Geometry check sheet. Reference: the model listing, model coordinates, mm. A direction names the side the tool comes from. Give positions to 0.01 mm unless a question says otherwise; leave off trailing zeros. Loops run counter-clockwise (first coordinate to the right, second up) from the corner with the lowest first, then second, coordinate; pieces in that order, holes last. Notation, with made-up numbers: (28.25, 35.5) -> (36.25, 35.5) arc R29 ccw to (36.25, 64.5) -> close; hole circle Ø5 at (8, 32.25). An arc over 180 degrees is marked (long way). One line per item, written item: value. Start each with the question number.
(1) Gauge pin test, flat ends, axial feed: pin 1 Ø3 at (x, z) = (-11, 15) entering from +Y; pin 2 Ø3 at (x, y) = (9.5, 0) entering from +Z. Record the tip position at first contact, or that the pin passes through.
(2) Scan lines: line 1 along X through (y, z) = (-16.75, 13.7); line 2 along Y through (x, z) = (9.25, 18.5); line 3 along Z through (x, y) = (-3.25, -3). Record each from-to range of solid material in increasing order. Write a range as from..to.
(3) Tool access check on faces 1 (the face through (10.31, -0.34, 1.82)), 2 (the face through (0, 0, 3.7)), 3 (the face through (0, -17, 34.95)). Record the directions out of +Z, -Z, +X, -X, +Y, -Y that give a thin tool (end or side, any length) a straight path to the whole face; none if there is none.
(4) Draft check along Y on faces 4 (the face through (-7, -16, 28)), 5 (the face through (15, -16.4, 17)), 6 (the face through (-4.34, 7.45, 1.82)). Enter one of: pulls with the +Y half, pulls with the -Y half, needs draft (parallel to the pull), parting line crosses it, or undercut.
(5) Sectioned sample at C-C, the plane z = 43. Record the cut outline in (x, y), then the cut area to 3 significant figures.
(6) Sectioned sample at A-A, the plane z = 16.5. Record the cut outline in (x, y).
(7) Sectioned sample at B-B, the plane x = 4.75. Record the cut outline in (y, z), then the cut area to 3 significant figures.
(8) Sectioned sample at D-D, the plane x = -2. Record the cut outline in (y, z).
from build123d import *

# Parameters (mm, degrees)
SKETCH_1_R      = 0.88
EXTRUDE_1_DEPTH = 3.7
SKETCH_3_W      = 30
SKETCH_3_H      = 50
SKETCH_3_R      = 1.65
SKETCH_3_R_2    = 1.1
EXTRUDE_2_DEPTH = 2


with BuildPart() as part:
    # 草图1 → 凸台-拉伸1 (new body)
    with BuildSketch(Plane.XY):
        with BuildLine():
            Line((-15, 0), (-15, -18))
            Line((-15, -18), (15, -18))
            Line((15, -18), (15, 0))
            ThreePointArc((15, 0), (0, 15), (-15, 0))
        make_face()
        with Locations((9.5, 0)):
            Circle(SKETCH_1_R, mode=Mode.SUBTRACT)
        with Locations((4.75, -8.227241336)):
            Circle(SKETCH_1_R, mode=Mode.SUBTRACT)
        with Locations((-4.75, -8.227241336)):
            Circle(SKETCH_1_R, mode=Mode.SUBTRACT)
        with Locations((-9.5, 0)):
            Circle(SKETCH_1_R, mode=Mode.SUBTRACT)
        with Locations((-4.75, 8.227241336)):
            Circle(SKETCH_1_R, mode=Mode.SUBTRACT)
        with Locations((4.75, 8.227241336)):
            Circle(SKETCH_1_R, mode=Mode.SUBTRACT)
    extrude(amount=EXTRUDE_1_DEPTH)

    # 草图3 → 凸台-拉伸2 (add)
    with BuildSketch(Plane(origin=(0, -18, 0), x_dir=(1, 0, 0), z_dir=(0, 1, 0))):
        with Locations((0, -28.7)):
            Rectangle(SKETCH_3_W, SKETCH_3_H)
        with Locations(Location((-10, -13.7, 0), (0, 0, 270))):
            Circle(SKETCH_3_R, mode=Mode.SUBTRACT)
        with Locations(Location((10, -13.7, 0), (0, 0, 90))):
            Circle(SKETCH_3_R, mode=Mode.SUBTRACT)
        with Locations(Location((10, -43.7, 0), (0, 0, 270))):
            Circle(SKETCH_3_R, mode=Mode.SUBTRACT)
        with Locations(Location((-10, -43.7, 0), (0, 0, 90))):
            Circle(SKETCH_3_R, mode=Mode.SUBTRACT)
        with Locations(Location((0, -8.95, 0), (0, 0, 270))):
            Circle(SKETCH_3_R_2, mode=Mode.SUBTRACT)
        with Locations(Location((0, -37.95, 0), (0, 0, 270))):
            Circle(SKETCH_3_R_2, mode=Mode.SUBTRACT)
        Polygon((-6.25, -28.7), (-6.25, -11.95), (6.25, -11.95), (6.25, -28.7), (6.25, -34.95), (-6.25, -34.95), align=None, mode=Mode.SUBTRACT)
    extrude(amount=EXTRUDE_2_DEPTH)


solid = part.part
Calculated:
1. pin 1: stops at y = -16
1. pin 2: stops at z = 3.7
2. line 1: x = -15..-11.65, -8.35..-6.25, 6.25..8.35, 11.65..15
2. line 2: y = -18..-16
2. line 3: z = 0..3.7
3. face 1: +Z, -Z
3. face 2: +Z, +X, -X, +Y
3. face 3: +Y, -Y
4. face 4: pulls with the +Y half
4. face 5: needs draft
4. face 6: undercut
5. outline: (-15, -18) -> (-11.49, -18) -> (-11.49, -16) -> (-15, -16) -> close; (-8.51, -18) -> (8.51, -18) -> (8.51, -16) -> (-8.51, -16) -> close; (11.49, -18) -> (15, -18) -> (15, -16) -> (11.49, -16) -> close
5. area: 48.0 mm2
6. outline: (-15, -18) -> (-6.25, -18) -> (-6.25, -16) -> (-15, -16) -> close; (6.25, -18) -> (15, -18) -> (15, -16) -> (6.25, -16) -> close
7. outline: (-18, 0) -> (-9.11, 0) -> (-9.11, 3.7) -> (-16, 3.7) -> (-16, 11.95) -> (-18, 11.95) -> close; (-18, 34.95) -> (-16, 34.95) -> (-16, 53.7) -> (-18, 53.7) -> close; (-7.35, 0) -> (7.35, 0) -> (7.35, 3.7) -> (-7.35, 3.7) -> close; (9.11, 0) -> (14.23, 0) -> (14.23, 3.7) -> (9.11, 3.7) -> close
7. area: 160 mm2
8. outline: (-18, 0) -> (14.87, 0) -> (14.87, 3.7) -> (-16, 3.7) -> (-16, 11.95) -> (-18, 11.95) -> close; (-18, 34.95) -> (-16, 34.95) -> (-16, 53.7) -> (-18, 53.7) -> close
